Geometry check sheet. Reference: drawing and pictorial views, mm from the part's lowest x, y, z. Round coordinates to 2 decimals unless told otherwise and drop trailing zeros. Loops run counter-clockwise (first coordinate to the right, second up) from the corner with the lowest first, then second, coordinate; pieces in that order, holes last. Notation, with made-up numbers: (76.25, -31) -> (95.25, -31) arc R13 cw to (95.25, -11) -> close; hole circle Ø7 at (4, 51). An arc over 180 degrees is marked (long way). Write item = value, one per line.
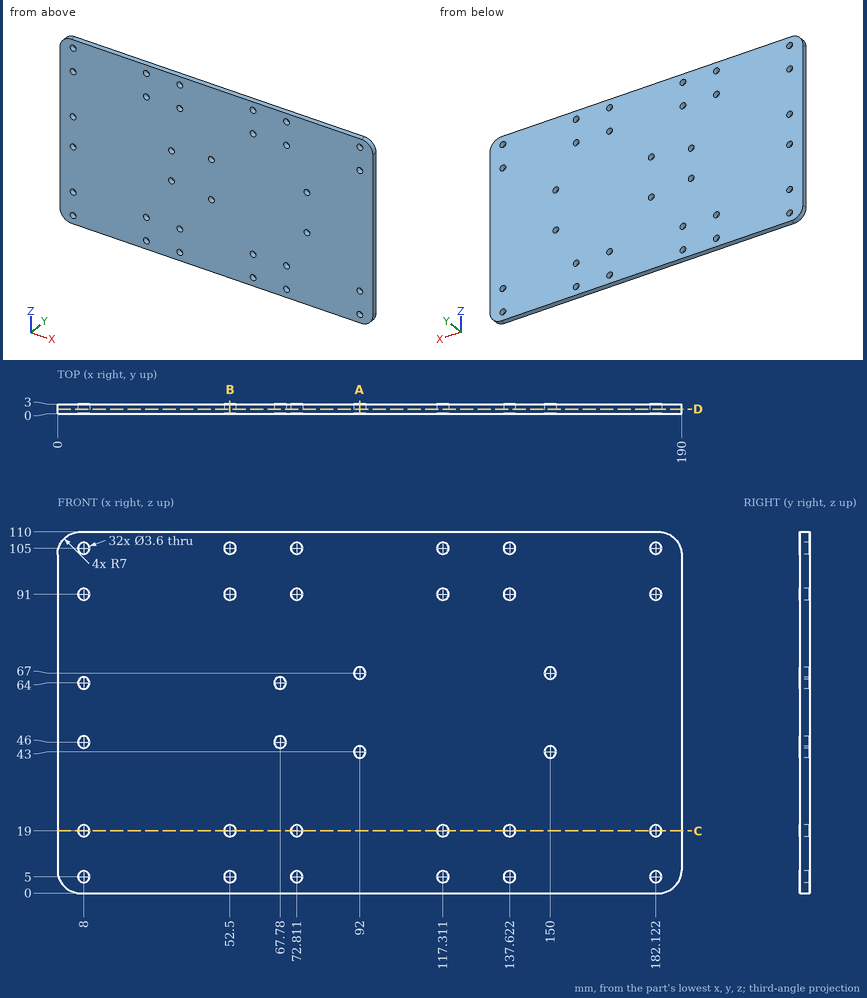
(1) Sectioned sample at C-C, the plane z = 19. Record the cut outline in (x, y), and give its area (3 significant figures).
Filled sheet:
outline = (0, 0) -> (6.2, 0) -> (6.2, 3) -> (0, 3) -> close; (9.8, 0) -> (50.7, 0) -> (50.7, 3) -> (9.8, 3) -> close; (54.3, 0) -> (71.01, 0) -> (71.01, 3) -> (54.3, 3) -> close; (74.61, 0) -> (115.51, 0) -> (115.51, 3) -> (74.61, 3) -> close; (119.11, 0) -> (135.82, 0) -> (135.82, 3) -> (119.11, 3) -> close; (139.42, 0) -> (180.32, 0) -> (180.32, 3) -> (139.42, 3) -> close; (183.92, 0) -> (190, 0) -> (190, 3) -> (183.92, 3) -> close
area = 505 mm2
(2) Sectioned sample at D-D, the plane y = 1.45. Count the separate pieces of the cut face and the enclosed holes in it, and give its area (3 significant figures).
Filled sheet:
separate_pieces = 1
enclosed_holes = 32
area = 20,500 mm2
(3) Sectioned sample at A-A, the plane x = 92. Record the cut outline in (y, z), and give its area (3 significant figures).
Filled sheet:
outline = (0, 0) -> (3, 0) -> (3, 41.2) -> (0, 41.2) -> close; (0, 44.8) -> (3, 44.8) -> (3, 65.2) -> (0, 65.2) -> close; (0, 68.8) -> (3, 68.8) -> (3, 110) -> (0, 110) -> close
area = 308 mm2
(4) Material ranges on probe 1 along X at (y, z) = (2.8, 43); probe 2 along Z at (x, y) = (150, 0.95); probe 3 along Z at (x, y) = (67.78, 1.35), recorded low to high. Write a range as from..to.
Filled sheet:
probe_1 = 0..90.2, 93.8..148.2, 151.8..190
probe_2 = 0..41.2, 44.8..65.2, 68.8..110
probe_3 = 0..44.2, 47.8..62.2, 65.8..110
(5) Sectioned sample at B-B, the plane x = 52.5. Record the cut outline in (y, z).
Filled sheet:
outline = (0, 0) -> (3, 0) -> (3, 3.2) -> (0, 3.2) -> close; (0, 6.8) -> (3, 6.8) -> (3, 17.2) -> (0, 17.2) -> close; (0, 20.8) -> (3, 20.8) -> (3, 89.2) -> (0, 89.2) -> close; (0, 92.8) -> (3, 92.8) -> (3, 103.2) -> (0, 103.2) -> close; (0, 106.8) -> (3, 106.8) -> (3, 110) -> (0, 110) -> close
